Can you work these out from the model? Positions are in its coordinate system, mm. A direction names the side the tool comes from. Give positions to 0.01 mm unless a question says otherwise; leave off trailing zeros. Loops run counter-clockwise (first coordinate to the right, second up) from the corner with the lowest first, then second, coordinate; pieces in that order, holes last. Notation, with made-up numbers: (59.5, 77.25) -> (77.5, 77.25) arc R8 cw to (77.5, 92.25) -> close; hole circle Ø3 at (60.25, -12). An arc over 180 degrees is marked (long way). One line per question, with ' | ' between items.
from build123d import *

# Parameters (mm, degrees)
SKETCH1_W           = 35.56
SKETCH1_H           = 10.16
BOSS_EXTRUDE1_DEPTH = 2.8
SKETCH3_R           = 0.915
CUT_EXTRUDE1_DEPTH  = 0.78
SKETCH4_W           = 35.56
SKETCH4_H           = 5.08
CUT_EXTRUDE2_DEPTH  = 0.8
SKETCH5_R           = 2.25
SKETCH5_W           = 13.4325
SKETCH5_H           = 5.08
CUT_EXTRUDE3_DEPTH  = 3
SKETCH6_R           = 0.71
CUT_EXTRUDE4_DEPTH  = 3.02


with BuildPart() as part:
    # Sketch1 → Boss-Extrude1 (new body)
    with BuildSketch(Plane(origin=(0, 0, 0), x_dir=(1, 0, 0), z_dir=(0, 1, 0))):
        with Locations((17.78, 5.08)):
            Rectangle(SKETCH1_W, SKETCH1_H)
    extrude(amount=BOSS_EXTRUDE1_DEPTH)

    # Sketch3 → Cut-Extrude1 (cut)
    with BuildSketch(Plane(origin=(0, 2.8, 0), x_dir=(1, 0, 0), z_dir=(0, 1, 0))):
        with Locations((1.27, 8.89)):
            Circle(SKETCH3_R)
        with Locations((3.81, 8.89)):
            Circle(SKETCH3_R)
        with Locations((6.35, 8.89)):
            Circle(SKETCH3_R)
        with Locations((8.89, 8.89)):
            Circle(SKETCH3_R)
        with Locations((11.43, 8.89)):
            Circle(SKETCH3_R)
        with Locations((13.97, 8.89)):
            Circle(SKETCH3_R)
        with Locations((16.51, 8.89)):
            Circle(SKETCH3_R)
        with Locations((19.05, 8.89)):
            Circle(SKETCH3_R)
        with Locations((21.59, 8.89)):
            Circle(SKETCH3_R)
        with Locations((24.13, 8.89)):
            Circle(SKETCH3_R)
        with Locations((26.67, 8.89)):
            Circle(SKETCH3_R)
        with Locations((29.21, 8.89)):
            Circle(SKETCH3_R)
        with Locations((31.75, 8.89)):
            Circle(SKETCH3_R)
        with Locations((34.29, 8.89)):
            Circle(SKETCH3_R)
        with Locations((3.81, 1.27)):
            Circle(SKETCH3_R)
        with Locations((6.35, 1.27)):
            Circle(SKETCH3_R)
        with Locations((8.89, 1.27)):
            Circle(SKETCH3_R)
        with Locations((11.43, 1.27)):
            Circle(SKETCH3_R)
        with Locations((13.97, 1.27)):
            Circle(SKETCH3_R)
        with Locations((16.51, 1.27)):
            Circle(SKETCH3_R)
        with Locations((19.05, 1.27)):
            Circle(SKETCH3_R)
        with Locations((21.59, 1.27)):
            Circle(SKETCH3_R)
        with Locations((24.13, 1.27)):
            Circle(SKETCH3_R)
        with Locations((26.67, 1.27)):
            Circle(SKETCH3_R)
        with Locations((29.21, 1.27)):
            Circle(SKETCH3_R)
        with Locations((31.75, 1.27)):
            Circle(SKETCH3_R)
        with Locations((34.29, 1.27)):
            Circle(SKETCH3_R)
        with Locations((1.27, 1.27)):
            Circle(SKETCH3_R)
    extrude(amount=-CUT_EXTRUDE1_DEPTH, mode=Mode.SUBTRACT)

    # Sketch4 → Cut-Extrude2 (cut)
    with BuildSketch(Plane(origin=(0, 2.8, 0), x_dir=(1, 0, 0), z_dir=(0, 1, 0))):
        with Locations((17.78, 5.08)):
            Rectangle(SKETCH4_W, SKETCH4_H)
    extrude(amount=-CUT_EXTRUDE2_DEPTH, mode=Mode.SUBTRACT)

    # Sketch5 → Cut-Extrude3 (cut, through all)
    with BuildSketch(Plane(origin=(0, 2, 0), x_dir=(1, 0, 0), z_dir=(0, 1, 0))):
        with Locations((-0.98, 5.08)):
            Circle(SKETCH5_R)
        with Locations((9.61125, 5.08)):
            Rectangle(SKETCH5_W, SKETCH5_H)
        with Locations((25.94375, 5.08)):
            Rectangle(SKETCH5_W, SKETCH5_H)
    extrude(amount=-CUT_EXTRUDE3_DEPTH, mode=Mode.SUBTRACT)

    # Sketch6 → Cut-Extrude4 (cut, through all)
    with BuildSketch(Plane(origin=(0, 2.02, 0), x_dir=(1, 0, 0), z_dir=(0, 1, 0))):
        with Locations((1.27, 8.89)):
            Circle(SKETCH6_R)
        with Locations((3.81, 8.89)):
            Circle(SKETCH6_R)
        with Locations((6.35, 8.89)):
            Circle(SKETCH6_R)
        with Locations((8.89, 8.89)):
            Circle(SKETCH6_R)
        with Locations((11.43, 8.89)):
            Circle(SKETCH6_R)
        with Locations((13.97, 8.89)):
            Circle(SKETCH6_R)
        with Locations((16.51, 8.89)):
            Circle(SKETCH6_R)
        with Locations((19.05, 8.89)):
            Circle(SKETCH6_R)
        with Locations((21.59, 8.89)):
            Circle(SKETCH6_R)
        with Locations((24.13, 8.89)):
            Circle(SKETCH6_R)
        with Locations((26.67, 8.89)):
            Circle(SKETCH6_R)
        with Locations((29.21, 8.89)):
            Circle(SKETCH6_R)
        with Locations((31.75, 8.89)):
            Circle(SKETCH6_R)
        with Locations((34.29, 8.89)):
            Circle(SKETCH6_R)
        with Locations((3.81, 1.27)):
            Circle(SKETCH6_R)
        with Locations((6.35, 1.27)):
            Circle(SKETCH6_R)
        with Locations((8.89, 1.27)):
            Circle(SKETCH6_R)
        with Locations((11.43, 1.27)):
            Circle(SKETCH6_R)
        with Locations((13.97, 1.27)):
            Circle(SKETCH6_R)
        with Locations((16.51, 1.27)):
            Circle(SKETCH6_R)
        with Locations((19.05, 1.27)):
            Circle(SKETCH6_R)
        with Locations((21.59, 1.27)):
            Circle(SKETCH6_R)
        with Locations((24.13, 1.27)):
            Circle(SKETCH6_R)
        with Locations((26.67, 1.27)):
            Circle(SKETCH6_R)
        with Locations((29.21, 1.27)):
            Circle(SKETCH6_R)
        with Locations((31.75, 1.27)):
            Circle(SKETCH6_R)
        with Locations((34.29, 1.27)):
            Circle(SKETCH6_R)
        with Locations((1.27, 1.27)):
            Circle(SKETCH6_R)
    extrude(amount=-CUT_EXTRUDE4_DEPTH, mode=Mode.SUBTRACT)


solid = part.part
Q1. On a 3-axis mill with a long thin cutter (end or side, diameter ignored), from which of +Z, -Z, +X, -X, +Y, -Y can I reach the whole of each face in a straight line? I mean faces 1 (the face through (34, 2, -5)), 2 (the face through (32.595, 2.415, -0.92)), 3 (the face through (2.895, 1, -5)). Say none if no direction works.
Entries:
face 1: +X, -X, +Y | face 2: +Y | face 3: +Y, -Y
Q2. If we section it at A-A (x = 6.35): Write out the boundary of the cut face in (y, z) (3 decimals).
Entries:
outline: (0, -10.16) -> (2.8, -10.16) -> (2.8, -9.805) -> (2.02, -9.805) -> (2.02, -9.6) -> (0, -9.6) -> close; (0, -8.18) -> (2.02, -8.18) -> (2.02, -7.975) -> (2.8, -7.975) -> (2.8, -7.62) -> (0, -7.62) -> close; (0, -2.54) -> (2.8, -2.54) -> (2.8, -2.185) -> (2.02, -2.185) -> (2.02, -1.98) -> (0, -1.98) -> close; (0, -0.56) -> (2.02, -0.56) -> (2.02, -0.355) -> (2.8, -0.355) -> (2.8, 0) -> (0, 0) -> close
Q3. For pin 1 Ø1.5 at (x, z) = (34.5, -1.5) entering from +Y; pin 2 Ø1.1 at (x, z) = (24.13, -1.27) entering from +Y; pin 3 Ø1.5 at (x, z) = (6.35, -8.89) entering from +Y, each with a flat end and sliding along its axis, tell me the tip position at first contact or that it passes through.
Entries:
pin 1: y = 2.8 | pin 2: through | pin 3: y = 2.02
Q4. If we section it at B-B (z = -4.25): Write out the boundary of the cut face in (x, y) (1 decimal), plus the area to 3 significant figures.
Entries:
outline: (1.1, 0) -> (2.9, 0) -> (2.9, 2) -> (1.1, 2) -> close; (16.3, 0) -> (19.2, 0) -> (19.2, 2) -> (16.3, 2) -> close; (32.7, 0) -> (35.6, 0) -> (35.6, 2) -> (32.7, 2) -> close | area: 15.2 mm²
Q5. If we mould it in two halves opening along X, with no side actions, what happens to faces 4 (the face through (18, 1, -10.16)), 5 (the face through (27.515, 2.415, -8.54))? For each: pulls with the +X half, pulls with the -X half, needs draft (parallel to the pull), parting line crosses it, or undercut.
Entries:
face 4: needs draft | face 5: undercut
Q6. If we section it at C-C (x = 34.29): Write out the boundary of the cut face in (y, z) (3 decimals), plus the area to 3 significant figures.
Entries:
outline: (0, -10.16) -> (2.8, -10.16) -> (2.8, -9.805) -> (2.02, -9.805) -> (2.02, -9.6) -> (0, -9.6) -> close; (0, -8.18) -> (2.02, -8.18) -> (2.02, -7.975) -> (2.8, -7.975) -> (2.8, -7.62) -> (2, -7.62) -> (2, -2.54) -> (2.8, -2.54) -> (2.8, -2.185) -> (2.02, -2.185) -> (2.02, -1.98) -> (0, -1.98) -> close; (0, -0.56) -> (2.02, -0.56) -> (2.02, -0.355) -> (2.8, -0.355) -> (2.8, 0) -> (0, 0) -> close | area: 15.8 mm²
Q7. If we section it at D-D (y = 2.4): State how many separate pieces and enclosed holes the cut face has, plus the area to 3 significant figures.
Entries:
separate pieces: 2 | enclosed holes: 28 | area: 107 mm²
Q8. If I drill on probe 1 along X at (y, z) = (1.8, -3) (1 decimal); probe 2 along Z at (x, y) = (13.97, 0.95); probe 3 along Z at (x, y) = (19.05, 2.3) (3 decimals), over which ranges is the centre line in solid material (lowest first)? Write a range as from..to.
Entries:
probe 1: 0..2.9, 16.3..19.2, 32.7..35.6 | probe 2: -10.16..-9.6, -8.18..-7.62, -2.54..-1.98, -0.56..0 | probe 3: -10.16..-9.805, -7.975..-7.62, -2.54..-2.185, -0.355..0
